from build123d import *

# Parameters (mm, degrees)
F1_DEPTH = 44
F2_R     = 3
F3_DEPTH = 3
F4_W     = 21.4669842049
F4_H     = 12
F5_DEPTH = 3
F6_R     = 3
F6_R_2   = 2.5
F7_DEPTH = 25


with BuildPart() as f1:
    # F0 (on Right) → F1 (new body)
    with BuildSketch(Plane.YZ):
        Polygon((6, -20), (6, 20), (3, 20), (3, -17), (-3, -17), (-3, 20), (-6, 20), (-6, -20), align=None)
    extrude(amount=F1_DEPTH)

    # F2 (on face) → F3 (join)
    with BuildSketch(Plane(origin=(0, 0, 0), x_dir=(0, -1, 0), z_dir=(-1, 0, 0))):
        with BuildLine():
            Line((-3, -17), (-3, 20))
            Line((-3, 20), (-18, 20))
            ThreePointArc((-18, 20), (-21.5355339059, 18.5355339059), (-23, 15))
            Line((-23, 15), (-23, -12))
            ThreePointArc((-23, -12), (-21.5355339059, -15.5355339059), (-18, -17))
            Line((-18, -17), (-3, -17))
        make_face()
        with Locations((-16, -10)):
            Circle(F2_R, mode=Mode.SUBTRACT)
        with Locations((-16, 13)):
            Circle(F2_R, mode=Mode.SUBTRACT)
        with BuildLine():
            Line((18, 20), (3, 20))
            Line((3, 20), (3, -17))
            Line((3, -17), (18, -17))
            ThreePointArc((18, -17), (21.5355339059, -15.5355339059), (23, -12))
            Line((23, -12), (23, 15))
            ThreePointArc((23, 15), (21.5355339059, 18.5355339059), (18, 20))
        make_face()
        with Locations((16, -10)):
            Circle(F2_R, mode=Mode.SUBTRACT)
        with Locations((16, 13)):
            Circle(F2_R, mode=Mode.SUBTRACT)
    extrude(amount=F3_DEPTH)

    # F4 (on face) → F5 (cut)
    with BuildSketch(Plane(origin=(0, 0, -20), x_dir=(1, 0, 0), z_dir=(0, 0, -1))):
        with Locations((33.2665078975, 0)):
            Rectangle(F4_W, F4_H)
    extrude(amount=-F5_DEPTH, mode=Mode.SUBTRACT)

    # F6 (on face) → F7 (cut)
    with BuildSketch(Plane(origin=(0, 6, 0), x_dir=(-1, 0, 0), z_dir=(0, 1, 0))):
        with BuildLine():
            Line((-44, -17), (-37, -17))
            Line((-37, -17), (-37, 8))
            ThreePointArc((-37, 8), (-37.5857864376, 9.4142135624), (-39, 10))
            Line((-39, 10), (-42, 10))
            ThreePointArc((-42, 10), (-43.4142135624, 10.5857864376), (-44, 12))
            Line((-44, 12), (-44, -17))
        make_face()
        with Locations((-39, 15)):
            Circle(F6_R)
        with BuildLine():
            Line((-44, 20), (-44, 18))
            ThreePointArc((-44, 18), (-43.4142135624, 19.4142135624), (-42, 20))
            Line((-42, 20), (-44, 20))
        make_face()
        with BuildLine():
            Line((-2, -19), (-2, -20))
            Line((-2, -20), (0, -20))
            Line((0, -20), (0, -17))
            ThreePointArc((0, -17), (-1.4142135624, -17.5857864376), (-2, -19))
        make_face()
        with BuildLine():
            add(Edge.make_bspline(
                [(-22.5330157951, -17), (-22.7836436775, -16.1303906467), (-23.1942051069, -14.7058546262), (-24.5152526704, -14.1009978001), (-26.3186845718, -15.8337712078), (-27.5330157951, -17)],
                knots=[0, 0, 0, 0, 0.3386124105, 0.5546847127, 1, 1, 1, 1], degree=3))
            Line((-27.5330157951, -17), (-22.5330157951, -17))
        make_face()
        with Locations((-18, -7)):
            Circle(F6_R_2)
    extrude(amount=-F7_DEPTH, mode=Mode.SUBTRACT)


solid = f1.part
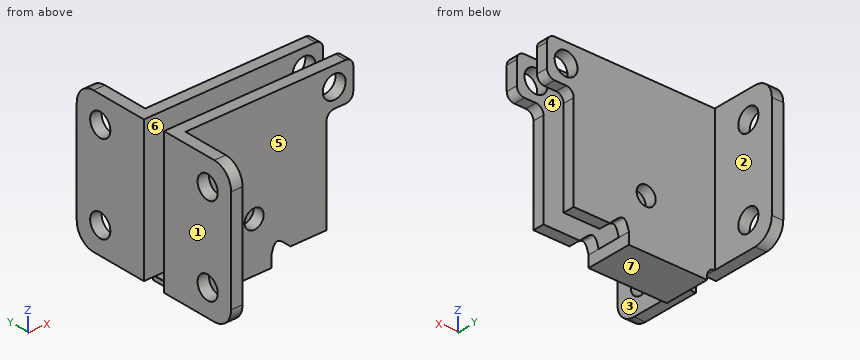
The listing builds one solid part. Answer for the finished solid, in the listing's coordinates (mm). Face numbers are marked on the shaded views. A direction names the side the tool comes from. Give positions to 0.01 mm unless a question says otherwise; leave off trailing zeros. Loops run counter-clockwise (first coordinate to the right, second up) from the corner with the lowest first, then second, coordinate; pieces in that order, holes last. Notation, with made-up numbers: M 14.25,87 L 20.25,87 A25 cw 20.25,102 Z; hole C 34.5,70 d9. An arc over 180 degrees is marked long. Answer as CSV lines item,"result".
Item 1: Which of the six approach directions +Z, -Z, +X, -X, +Y, -Y give full straight-line access (tool end or side, diameter ignored) to the marked faces 1, 2 and 3?
Values follow:
face 1,"+Z, -Z, -X, +Y, -Y"
face 2,"+Z, -Z, +X, +Y"
face 3,"+Z, -Z, +X, -Y"
Item 2: The part is cut by section A-A (y = 16). Give the vertices of the cut face in (x, z).
Values follow:
outline,"M -3,-17 L 0,-17 L 0,-13 L -3,-13 Z; M -3,-7 L 0,-7 L 0,10 L -3,10 Z; M -3,16 L 0,16 L 0,20 L -3,20 Z"
Item 3: Straight lines are drawn through the part: line 1 along Z through (x, y) = (-1.6, 16); line 2 along Z through (x, y) = (18, -3.85); line 3 along Y through (x, z) = (19.5, 13). For each, find the intervals that lie inside material, in ascending order. Write a range as [from, to].
Values follow:
line 1,"z = [-17, -13], [-7, 10], [16, 20]"
line 2,"z = [-20, -9.5], [-4.5, 20]"
line 3,"y = [-6, -3], [3, 6]"
Item 4: The mould has two halves that part along Y. Classify the marked faces 4, 5, 6 and 7: released by +Y, released by -Y, zero draft, split by the parting line, or undercut.
Values follow:
face 4,"undercut"
face 5,"released by -Y"
face 6,"undercut"
face 7,"zero draft"
Item 5: Given pin 1 Ø8 at (x, z) = (18, -7) entering from -Y; pin 2 Ø2.5 at (x, y) = (-1, 11) entering from -Z; pin 3 Ø4 at (x, z) = (17, -9) entering from +Y, each flat-ended and moving along its own axis, determine where each tip first touches the part or whether it passes through.
Values follow:
pin 1,"stops at y = -6"
pin 2,"stops at z = -17"
pin 3,"stops at y = 6"
Item 6: The part is cut by section B-B (x = 31). Give the vertices of the cut face in (y, z), and give its area (3 significant figures).
Values follow:
outline,"M -6,-17 L -3,-17 L -3,20 L -6,20 Z; M 3,-17 L 6,-17 L 6,20 L 3,20 Z"
area,"222 mm^2"
Item 7: The part is cut by section D-D (z = 17). Give the vertices of the cut face in (x, y), and give its area (3 significant figures).
Values follow:
outline,"M -3,-22.58 L 0,-22.58 L 0,-6 L 36.76,-6 L 36.76,-3 L -3,-3 Z; M -3,3 L 36.76,3 L 36.76,6 L 0,6 L 0,22.58 L -3,22.58 Z; M 41.24,-6 L 44,-6 L 44,-3 L 41.24,-3 Z; M 41.24,3 L 44,3 L 44,6 L 41.24,6 Z"
area,"355 mm^2"
Item 8: The part is cut by section C-C (x = 18). Give the vertices of the cut face in (y, z), and give its area (3 significant figures).
Values follow:
outline,"M -6,-20 L 6,-20 L 6,-9.5 L 3,-9.5 L 3,-17 L -3,-17 L -3,-9.5 L -6,-9.5 Z; M -6,-4.5 L -3,-4.5 L -3,20 L -6,20 Z; M 3,-4.5 L 6,-4.5 L 6,20 L 3,20 Z"
area,"228 mm^2"
